```python
from build123d import *

# Parameters (mm, degrees)
CYLINDER019_R          = 1.6
CYLINDER019_DEPTH      = 10
PRISM002_DEPTH         = 3
BOX022_W               = 10
BOX022_H               = 11
BOX022_DEPTH           = 7
CYLINDER020_R          = 1.6
CYLINDER020_DEPTH      = 10
PRISM003_DEPTH         = 3
BOX023_W               = 8.5
BOX023_H               = 11
BOX023_DEPTH           = 7
CYLINDER017_R          = 1.6
CYLINDER017_DEPTH      = 10
CYLINDER017_ROLL_ANGLE = -90
CYLINDER015_R          = 1.6
CYLINDER015_DEPTH      = 10
CYLINDER015_ROLL_ANGLE = -90
BOX005_W               = 108
BOX005_H               = 3
BOX005_DEPTH           = 30
CHAMFER001_SIZE        = 1
CHAMFER002_SIZE        = 0.5
CHAMFER003_SIZE        = 0.5
CHAMFER003_ROLL_ANGLE  = -90


with BuildPart() as cylinder019:
    # Cylinder019 → Cylinder019 (new body)
    with BuildSketch(Plane(origin=(3.6, 5.69, -5), x_dir=(1, 0, 0), z_dir=(0, 0, 1))):
        Circle(CYLINDER019_R)
    extrude(amount=CYLINDER019_DEPTH)


with BuildPart() as prism002:
    # Prism002 → Prism002 (new body)
    with BuildSketch(Plane(origin=(3.6, 5.69, -7), x_dir=(1, 0, 0), z_dir=(0, 0, 1))):
        Polygon((3, 0), (1.5, 2.598076), (-1.5, 2.598076), (-3, 0), (-1.5, -2.598076), (1.5, -2.598076), align=None)
    extrude(amount=PRISM002_DEPTH)


with BuildPart() as cut010:
    # Box022 → Box022 (new body)
    with BuildSketch(Plane(origin=(-1.25, 0, -7), x_dir=(1, 0, 0), z_dir=(0, 0, 1))):
        with Locations((5, 5.5)):
            Rectangle(BOX022_W, BOX022_H)
    extrude(amount=BOX022_DEPTH)

    # Cut009: cut Prism002
    add(prism002.part, mode=Mode.SUBTRACT)


with BuildPart() as cut010_1:
    # Cut009 placement: moved
    add(cut010.part.moved(Location((0, 0, -1))))

    # Cut010: cut Cylinder019
    add(cylinder019.part, mode=Mode.SUBTRACT)


with BuildPart() as cut010_2:
    # Cut010 placement: moved
    add(cut010_1.part.moved(Location((0, 76.2, 0))))


with BuildPart() as cylinder020:
    # Cylinder020 → Cylinder020 (new body)
    with BuildSketch(Plane(origin=(3.6, 5.69, -5), x_dir=(1, 0, 0), z_dir=(0, 0, 1))):
        Circle(CYLINDER020_R)
    extrude(amount=CYLINDER020_DEPTH)


with BuildPart() as prism003:
    # Prism003 → Prism003 (new body)
    with BuildSketch(Plane(origin=(3.6, 5.69, -7), x_dir=(1, 0, 0), z_dir=(0, 0, 1))):
        Polygon((3, 0), (1.5, 2.598076), (-1.5, 2.598076), (-3, 0), (-1.5, -2.598076), (1.5, -2.598076), align=None)
    extrude(amount=PRISM003_DEPTH)


with BuildPart() as cut012:
    # Box023 → Box023 (new body)
    with BuildSketch(Plane(origin=(-1.25, 0, -7), x_dir=(1, 0, 0), z_dir=(0, 0, 1))):
        with Locations((4.25, 5.5)):
            Rectangle(BOX023_W, BOX023_H)
    extrude(amount=BOX023_DEPTH)

    # Cut011: cut Prism003
    add(prism003.part, mode=Mode.SUBTRACT)


with BuildPart() as cut012_1:
    # Cut011 placement: moved
    add(cut012.part.moved(Location((0, 0, -1))))

    # Cut012: cut Cylinder020
    add(cylinder020.part, mode=Mode.SUBTRACT)


with BuildPart() as cut012_2:
    # Cut012 placement: moved
    add(cut012_1.part.moved(Location((92.5, 76.2, 0))))


with BuildPart() as cylinder017:
    # Cylinder017 → Cylinder017 (new body)
    with BuildSketch(Plane.XY):
        Circle(CYLINDER017_R)
    extrude(amount=CYLINDER017_DEPTH)


with BuildPart() as cylinder017_1:
    # Cylinder017 roll: moved
    add(cylinder017.part.rotate(Axis((0, 0, 0), (1, 0, 0)), CYLINDER017_ROLL_ANGLE))


with BuildPart() as cylinder017_2:
    # Cylinder017 placement: moved
    add(cylinder017_1.part.moved(Location((96, 82, -18.7))))


with BuildPart() as left_holes:
    # Cylinder015 → Cylinder015 (new body)
    with BuildSketch(Plane.XY):
        Circle(CYLINDER015_R)
    extrude(amount=CYLINDER015_DEPTH)


with BuildPart() as left_holes_1:
    # Cylinder015 roll: moved
    add(left_holes.part.rotate(Axis((0, 0, 0), (1, 0, 0)), CYLINDER015_ROLL_ANGLE))


with BuildPart() as left_holes_2:
    # Cylinder015 placement: moved
    add(left_holes_1.part.moved(Location((3.6, 82, -18.7))))

    # Fusion006: union Cylinder017
    add(cylinder017_2.part)


with BuildPart() as left_side001:
    # Box005 → Box005 (new body)
    with BuildSketch(Plane(origin=(-5, 85, -25), x_dir=(1, 0, 0), z_dir=(0, 0, 1))):
        with Locations((54, 1.5)):
            Rectangle(BOX005_W, BOX005_H)
    extrude(amount=BOX005_DEPTH)

    # Cut026: cut left holes
    add(left_holes_2.part, mode=Mode.SUBTRACT)

    # Fusion012: union Cut010, Cut012
    add(cut010_2.part)
    add(cut012_2.part)

    # Chamfer001
    chamfer001_edges = [left_side001.edges().sort_by_distance(p)[0] for p in [
        (91.25, 85, -4.5),
        (8.75, 85, -4.5),
    ]]
    chamfer(chamfer001_edges, length=CHAMFER001_SIZE)

    # Chamfer002
    chamfer002_edges = [left_side001.edges().sort_by_distance(p)[0] for p in [
        (95.5, 85, -8),
    ]]
    chamfer(chamfer002_edges, length=CHAMFER002_SIZE)

    # Chamfer003
    chamfer003_edges = [left_side001.edges().sort_by_distance(p)[0] for p in [
        (3.75, 85, -8),
    ]]
    chamfer(chamfer003_edges, length=CHAMFER003_SIZE)


with BuildPart() as left_side001_1:
    # Chamfer003 roll: moved
    add(left_side001.part.rotate(Axis((0, 0, 0), (1, 0, 0)), CHAMFER003_ROLL_ANGLE))


with BuildPart() as left_side001_2:
    # Chamfer003 placement: moved
    add(left_side001_1.part.moved(Location((0, 123, 88))))


solid = left_side001_2.part
```
Work out the finished part from the listing and answer in its coordinate system (mm). A direction names the side the tool comes from. Round coordinates to 2 decimals unless told otherwise and drop trailing zeros. Write each loop counter-clockwise with the first axis right and the second up, starting at its lowest first coordinate (ties: lowest second). Pieces come first, ordered by that corner, then holes. Notation, with made-up numbers: (47.25, 3.25) - (68.25, 3.25) arc R6 ccw to (68.25, 10.25) - close; hole circle Ø9 at (11, -23). An arc over 180 degrees is marked (long way). Return JSON: item names as keys, results as strings. Group by question number.
Q1. The part is cut by section D-D on x = 82. Write down the section's boundary in (y, z).
Q2. Find the intervals of material crossed by L1, parallel to X at y = 120.7, z = 6.11; L2, parallel to Z at x = 96.1, y = 119.9; L3, parallel to Y at x = 96, z = 2, in increasing order.
Q3. The part is cut by section A-A on x = 3.6. Count the separate pieces of the cut face and the enclosed holes in it, then the cut area to 3 significant figures.
Q4. The part is cut by section B-B on y = 104.3. Write down the section's boundary in (x, z).
Q5. For faces 5 (the flat face through (97.4, 118, 4.9)), 6 (the flat face through (94, 115, 9)), 7 (the flat face through (91.25, 118, 8)), 8 (the flat face through (4, 118, 11.8)), determine the directions among +Z, -Z, +X, -X, +Y, -Y from which every point of the face is accessible in a straight line to the end or side of a thin tool.
Q6. Each of these flat-tipped pins is pushed along its axis until it touches: pin 1 Ø2 at (y, z) = (118.5, 8.5) entering from -X; pin 2 Ø4.5 at (x, z) = (97, 6.5) entering from +Y; pin 3 Ø4 at (y, z) = (119, 6.5) entering from +X; pin 4 Ø1.5 at (x, z) = (81.5, 4.5) entering from -Y. Where does it stop, or does it pass through?
Q7. The mould has two halves that part along X. Classify faces 1 (the cylindrical face through (3.392, 119.972, 4.524)), 2 (the flat face through (-5, 113, 2)), 3 (the flat face through (48, 98, 1)), 4 (the flat face through (98.34, 116.48, 7.43)): released by +X, released by -X, zero draft, split by the parting line, or undercut.
Solved:
{
 "1": {"outline": "(98, 0) - (128, 0) - (128, 3) - (98, 3) - close"},
 "2": {"L1": "-1.25 to 2, 5.2 to 8.75, 91.25 to 94.5, 97.7 to 99.75", "L2": "0 to 4.51, 7.71 to 11.8", "L3": "98 to 102.7, 105.9 to 128"},
 "3": {"separate pieces": "3", "enclosed holes": "0", "area": "114 mm²"},
 "4": {"outline": "(-5, 0) - (2, 0) - (2, 3) - (-5, 3) - close; (5.2, 0) - (94.4, 0) - (94.4, 3) - (5.2, 3) - close; (97.6, 0) - (103, 0) - (103, 3) - (97.6, 3) - close"},
 "5": {"face 5": "-Y", "face 6": "+Z, +X, -X, -Y", "face 7": "+Z, +Y, -Y", "face 8": "+Z, +X, -X, +Y, -Y"},
 "6": {"pin 1": "x = -1.25", "pin 2": "y = 122", "pin 3": "x = 99.75", "pin 4": "through"},
 "7": {"face 1": "undercut", "face 2": "released by -X", "face 3": "zero draft", "face 4": "undercut"}
}
